Part model, mm, in its own coordinate system. Face numbers are marked on the shaded views. A direction names the side the tool comes from. Round coordinates to 2 decimals unless told otherwise and drop trailing zeros. Write each loop counter-clockwise with the first axis right and the second up, starting at its lowest first coordinate (ties: lowest second). Pieces come first, ordered by that corner, then holes. Notation, with made-up numbers: (64.5, -23.5) -> (109.5, -23.5) arc R16 cw to (109.5, -5.5) -> close; hole circle Ø5 at (9.5, -18). An arc over 180 degrees is marked (long way). Return JSON: item names as keys, results as strings. Group by question number.
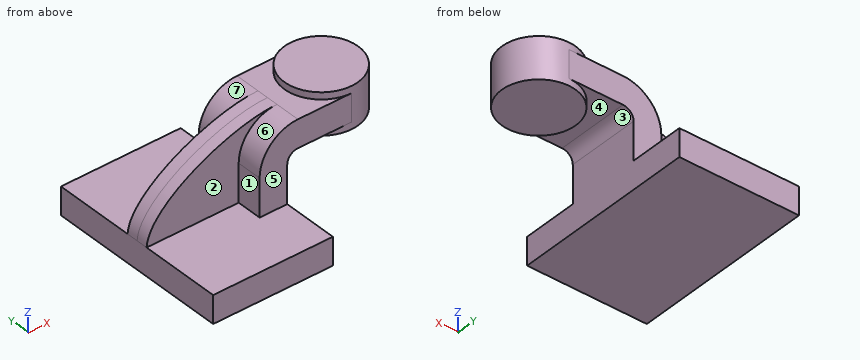
```python
from build123d import *

# Parameters (mm, degrees)
F1_DEPTH = 63.5
F0_W     = 25.4
F0_H     = 19.0500000358
F2_DEPTH = 25.4
F3_DEPTH = 7.9375


with BuildPart() as f1:
    # F0 (on Front) → F1 (new body, symmetric)
    with BuildSketch(Plane.XZ):
        Polygon((-41.275, -9.525), (41.275, -9.525), (41.275, 9.525), (22.2249999642, 9.525), (-41.275, 9.525), align=None)
    extrude(amount=F1_DEPTH, both=True)

    # F0 (on Front) → F2 (join, symmetric)
    with BuildSketch(Plane.XZ):
        with Locations((73.025, 52.4002000179)):
            Rectangle(F0_W, F0_H)
        with BuildLine():
            Line((22.2249999642, 9.525), (41.275, 9.525))
            Line((41.275, 9.525), (41.275, 35.5059314692))
            ThreePointArc((41.275, 35.5059314692), (43.4334087803, 40.7167912197), (48.6442685308, 42.8752))
            Line((48.6442685308, 42.8752), (60.325, 42.8752))
            Line((60.325, 42.8752), (60.325, 61.9252000358))
            Line((60.325, 61.9252000358), (48.6442685308, 61.9252000358))
            ThreePointArc((48.6442685308, 61.9252000358), (29.9630245734, 54.1871754266), (22.2249999642, 35.5059314692))
            Line((22.2249999642, 35.5059314692), (22.2249999642, 9.525))
        make_face()
    extrude(amount=F2_DEPTH, both=True)

    # F0 (on Front) → F3 (join, symmetric)
    with BuildSketch(Plane.XZ):
        with BuildLine():
            add(Edge.make_bspline(
                [(-41.275, 9.525), (-39.4913367927, 35.5950407684), (16.4129212499, 62.2470639646), (48.6442685308, 61.9252000358)],
                knots=[0, 0, 0, 0, 104.0733194287, 104.0733194287, 104.0733194287, 104.0733194287], degree=3))
            Line((-41.275, 9.525), (22.2249999642, 9.525))
            Line((22.2249999642, 9.525), (22.2249999642, 35.5059314692))
            ThreePointArc((22.2249999642, 35.5059314692), (29.9630245734, 54.1871754266), (48.6442685308, 61.9252000358))
        make_face()
    extrude(amount=F3_DEPTH, both=True)

    # F0 (on Front) → F4 (revolve)
    with BuildSketch(Plane.XZ):
        Polygon((85.725, 66.675), (85.725, 61.9252000358), (85.725, 42.8752), (85.725, 38.1), (111.125, 38.1), (111.125, 66.675), align=None)
    revolve(axis=Axis((85.725, 0, 52.3875), (0, 0, -1)))


solid = f1.part
```
Item 1: Cut at A-A (y = 18). Write the cut outline in (x, z) (3 decimals).
Item 2: Wall check: L1, parallel to Z at x = -27.5, y = 51 (3 decimals); L2, parallel to X at y = -53.5, z = 1 (3 decimals); L3, parallel to Y at x = 31.5, z = 36.5. Give the ranges that are in metal, low to high.
Item 3: Flat gauge pins, fed straight in: P1, Ø15.5, axis at x = 66.5, z = 42, coming from the -Y side; P2, Ø12, axis at x = -2, y = -33.5, coming from the +Z side (3 decimals); P3, Ø19, axis at y = 18, z = 22, coming from the -X side (3 decimals); P4, Ø10, axis at x = -11, z = 51.5, coming from the +Y side. Where does each tip first touch, or does it go through?
Item 4: Two-plate mould, pull along X, no slides. Class the marked faces 1, 2, 3 and 4: released by +X, released by -X, zero draft, split by the parting line, or undercut.
Item 5: Which spindle directions (+Z, -Z, +X, -X, +Y, -Y) get a long thin tool onto all of the face, cutting with end or side? Do the marked faces 5, 6 and 7. Say none if no direction does.
Item 6: Cut at B-B (z = 3). Write the cut outline in (x, y) (3 decimals).
Item 7: Cut at C-C (x = 56). Write the cut outline in (y, z), then the cut area to 3 significant figures.
Checks:
{
 "1": {"outline": "(-41.275, -9.525) -> (41.275, -9.525) -> (41.275, 35.506) arc R7.369 cw to (48.644, 42.875) -> (67.804, 42.875) -> (67.804, 38.1) -> (103.646, 38.1) -> (103.646, 66.675) -> (67.804, 66.675) -> (67.804, 61.925) -> (48.644, 61.925) arc R26.419 ccw to (22.225, 35.506) -> (22.225, 9.525) -> (-41.275, 9.525) -> close"},
 "2": {"L1": "z = -9.525 to 9.525", "L2": "x = -41.275 to 41.275", "L3": "y = -25.4 to 25.4"},
 "3": {"P1": "stops at y = -25.4", "P2": "stops at z = 9.525", "P3": "stops at x = 22.225", "P4": "passes through"},
 "4": {"face 1": "released by -X", "face 2": "zero draft", "face 3": "undercut", "face 4": "undercut"},
 "5": {"face 5": "+Z, +X, -X, -Y", "face 6": "+Z, -X, -Y", "face 7": "+Z, -X, +Y"},
 "6": {"outline": "(-41.275, -63.5) -> (41.275, -63.5) -> (41.275, 63.5) -> (-41.275, 63.5) -> close"},
 "7": {"outline": "(-25.4, 42.88) -> (25.4, 42.88) -> (25.4, 61.93) -> (-25.4, 61.93) -> close", "area": "968 mm2"}
}
